```python
from build123d import *

# Parameters (mm, degrees)
F0_W     = 63.5
F0_H     = 63.5
F0_R     = 25
F0_W_2   = 140
F0_H_2   = 60
F1_DEPTH = 6.35


# Not quite as in the source:
# - a length typed as a fraction of an inch, garbled in the dataset ("3 / 203.2 mm" for 3/8 in), is restored


with BuildPart() as f1:
    # F0 (on Right) → F1 (new body)
    with BuildSketch(Plane.YZ):
        Polygon((-400, -342.9), (450, -342.9), (450, 342.9), (-385, 342.9), (-450, 232.9), (-450, -277.9), align=None)
        with Locations((-360, -282.9)):
            Rectangle(F0_W, F0_H, mode=Mode.SUBTRACT)
        with Locations((-120, -282.9)):
            Rectangle(F0_W, F0_H, mode=Mode.SUBTRACT)
        with Locations((-380, -70)):
            Rectangle(F0_W, F0_H, mode=Mode.SUBTRACT)
        with Locations((-195, -70)):
            Rectangle(F0_W, F0_H, mode=Mode.SUBTRACT)
        with Locations((-10, -70)):
            Rectangle(F0_W, F0_H, mode=Mode.SUBTRACT)
        with Locations((120, -282.9)):
            Rectangle(F0_W, F0_H, mode=Mode.SUBTRACT)
        with Locations((360, -282.9)):
            Rectangle(F0_W, F0_H, mode=Mode.SUBTRACT)
        with Locations((175, -70)):
            Rectangle(F0_W, F0_H, mode=Mode.SUBTRACT)
        with Locations((360, -70)):
            Rectangle(F0_W, F0_H, mode=Mode.SUBTRACT)
        with Locations((-351.75, 60)):
            Rectangle(F0_W, F0_H, mode=Mode.SUBTRACT)
        with Locations((-141.75, 60)):
            Rectangle(F0_W, F0_H, mode=Mode.SUBTRACT)
        with Locations((-320, 272.9)):
            Rectangle(F0_W, F0_H, mode=Mode.SUBTRACT)
        with Locations((-150, 272.9)):
            Rectangle(F0_W, F0_H, mode=Mode.SUBTRACT)
        with Locations((68.25, 60)):
            Rectangle(F0_W, F0_H, mode=Mode.SUBTRACT)
        with Locations((278.25, 60)):
            Rectangle(F0_W, F0_H, mode=Mode.SUBTRACT)
        with Locations((395, 7.9)):
            Circle(F0_R, mode=Mode.SUBTRACT)
        with Locations((325, 152.9)):
            Rectangle(F0_W_2, F0_H_2, mode=Mode.SUBTRACT)
        with Locations((20, 272.9)):
            Rectangle(F0_W, F0_H, mode=Mode.SUBTRACT)
        with Locations((190, 272.9)):
            Rectangle(F0_W, F0_H, mode=Mode.SUBTRACT)
        with Locations((360, 272.9)):
            Rectangle(F0_W, F0_H, mode=Mode.SUBTRACT)
    extrude(amount=F1_DEPTH)


solid = f1.part
```
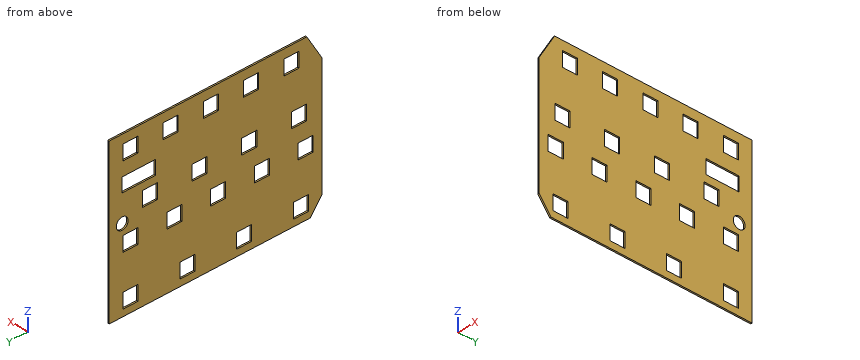
Part model, mm, in its own coordinate system. Coordinates: 2 decimals unless noted, no trailing zeros. Loops run counter-clockwise (first coordinate to the right, second up) from the corner with the lowest first, then second, coordinate; pieces in that order, holes last. Notation, with made-up numbers: (51.25, 51.5) - (101.25, 51.5) arc R16 cw to (101.25, 57.5) - close; hole circle Ø6 at (18.25, 62.5). An arc over 180 degrees is marked (long way). Write item = value, one per line. Start each with the question number.
Item 1: Cut at D-D, the plane x = 5. State how many separate pieces and enclosed holes the cut face has, and give its area (3 significant figures).
Item 2: Cut at B-B, the plane y = -302. Give the cut face in (x, z).
Item 3: Cut at A-A, the plane z = 7.9. Give the cut face in (x, y).
Item 4: Wall check: L1, parallel to Y at x = 0.75, z = 84.5; L2, parallel to Y at x = 1.25, z = -44; L3, parallel to Z at x = 3.25, y = 91.5. Give the ranges that are in metal, low to high. Write a range as from..to.
Item 5: Cut at C-C, the plane z = 292.5. Give the cut face in (x, y).
The answers:
q1.separate_pieces = 1
q1.enclosed_holes = 20
q1.area = 529,000 mm2
q2.outline = (0, -342.9) - (6.35, -342.9) - (6.35, 241.15) - (0, 241.15) - close; (0, 304.65) - (6.35, 304.65) - (6.35, 342.9) - (0, 342.9) - close
q3.outline = (0, -450) - (6.35, -450) - (6.35, 370) - (0, 370) - close; (0, 420) - (6.35, 420) - (6.35, 450) - (0, 450) - close
q4.L1 = -450..-383.5, -320..-173.5, -110..36.5, 100..246.5, 310..450
q4.L2 = -450..-411.75, -348.25..-226.75, -163.25..-41.75, 21.75..143.25, 206.75..328.25, 391.75..450
q4.L3 = -342.9..-314.65, -251.15..28.25, 91.75..342.9
q5.outline = (0, -414.78) - (6.35, -414.78) - (6.35, -351.75) - (0, -351.75) - close; (0, -288.25) - (6.35, -288.25) - (6.35, -181.75) - (0, -181.75) - close; (0, -118.25) - (6.35, -118.25) - (6.35, -11.75) - (0, -11.75) - close; (0, 51.75) - (6.35, 51.75) - (6.35, 158.25) - (0, 158.25) - close; (0, 221.75) - (6.35, 221.75) - (6.35, 328.25) - (0, 328.25) - close; (0, 391.75) - (6.35, 391.75) - (6.35, 450) - (0, 450) - close
